Verification items for the finished model (mm, model axes). Face numbers are marked on the shaded views. A direction names the side the tool comes from. Give positions to 0.01 mm unless a question says otherwise; leave off trailing zeros. Write each loop counter-clockwise with the first axis right and the second up, starting at its lowest first coordinate (ties: lowest second). Pieces come first, ordered by that corner, then holes. Notation, with made-up numbers: M 85,13 L 117,13 A17 ccw 117,18 Z; hole C -35,35 d9. An arc over 180 degrees is marked long. Answer as a JSON object with one key per item and string values.
```python
from build123d import *

# Parameters (mm, degrees)
SKETCH_2_W         = 6
SKETCH_2_H         = 2
HOLE_WIZARD_M3_1_D = 3.4


with BuildPart() as part:
    # 掃出1: sweep along a path in 草圖1
    with BuildLine(Plane.XY) as sweep_1_path:
        Line((-22, 2), (-11.832159566, 2))
        ThreePointArc((-11.832159566, 2), (0, 12), (11.832159566, 2))
        Line((11.832159566, 2), (22, 2))
    # 草圖2 → 掃出1 (sweep)
    with BuildSketch(Plane(origin=(22, 0, 0), x_dir=(0, 0, -1), z_dir=(1, 0, 0))):
        with Locations((0, 3)):
            Rectangle(SKETCH_2_W, SKETCH_2_H)
    sweep(path=sweep_1_path.line, transition=Transition.RIGHT)

    # M3 餘隙孔1 (through all)
    with Locations(Plane(origin=(0, 4, 0), x_dir=(1, 0, 0), z_dir=(0, 1, 0))):
        with Locations((-18, 0), (18, 0)):
            Hole(HOLE_WIZARD_M3_1_D / 2)


solid = part.part
```
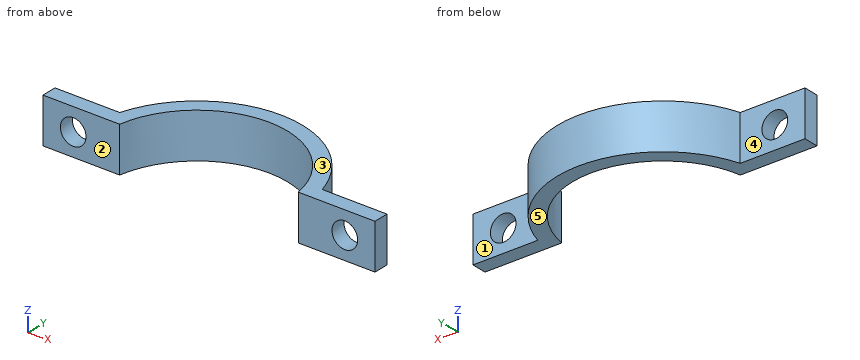
1) Thickness scan on L1, parallel to Z at x = 18, y = 2.4; L2, parallel to Y at x = -16.5, z = 2.5; L3, parallel to X at y = 10.5, z = 2.25. Record the ranges inside material, lowest first.
Completed:
{"L1": "z = -3 to -1.7, 1.7 to 3", "L2": "y = 2 to 4", "L3": "x = -9.26 to -5.81, 5.81 to 9.26"}
2) Section check B-B on z = 0. Count the separate pieces of the cut face and the enclosed holes in it, and give its area (3 significant figures).
Completed:
{"separate pieces": "3", "enclosed holes": "0", "area": "93.4 mm2"}
3) Access from +Z, -Z, +X, -X, +Y, -Y to the whole of each face (thin tool, end or side, straight path). Record for the marked faces 4 and 5.
Completed:
{"face 4": "+Z, -Z, -X, +Y", "face 5": "-Z, +X, -X, +Y, -Y"}
4) Go/stop test with flat-tipped pins: pin 1 (3 mm diameter, centred on x = 18, z = 0, fed in from -Y); pin 2 (1.8 mm diameter, centred on x = 17.5, z = 1.5, fed in from +Y). Record where each tip stops, or that it passes through.
Completed:
{"pin 1": "passes through", "pin 2": "stops at y = 4"}
5) Section check A-A on x = -18. Record the boundary of the cut face in (y, z).
Completed:
{"outline": "M 2,-3 L 4,-3 L 4,-1.7 L 2,-1.7 Z; M 2,1.7 L 4,1.7 L 4,3 L 2,3 Z"}
6) Release check for a two-part mould opening along Y. For the marked faces 1, 2 and 3 record: pulls with the +Y half, pulls with the -Y half, needs draft (parallel to the pull), parting line crosses it, or undercut.
Completed:
{"face 1": "pulls with the +Y half", "face 2": "pulls with the -Y half", "face 3": "needs draft"}
